Autodesk Inventor part; units mm, degrees
ref_plane "YZ Plane" through (0, 0, 0) normal (1, 0, 0) x (0, 1, 0)
ref_plane "XZ Plane" through (0, 0, 0) normal (0, 1, 0) x (-1, 0, 0)
ref_plane "XY Plane" through (0, 0, 0) normal (0, 0, 1) x (1, 0, 0)
sketch "Sketch1" plane through (0, 0, 0) normal (0, 0, 1) x (1, 0, 0)
  line L0 (-1.27, -1.27) -> (1.27, -1.27)
  line L1 (1.27, -1.27) -> (1.27, 1.27)
  line L2 (1.27, 1.27) -> (-1.27, 1.27)
  line L3 (-1.27, 1.27) -> (-1.27, -1.27)
  line L4 (-1.27, -1.27) -> (1.27, 1.27) construction
  line L5 (1.27, -1.27) -> (-1.27, 1.27) construction
  line L6 (-1.07, 1.07) -> (1.07, 1.07)
  line L7 (1.07, 1.07) -> (1.07, -1.07)
  line L8 (1.07, -1.07) -> (-1.07, -1.07)
  line L9 (-1.07, -1.07) -> (-1.07, 1.07)
  point P0 (0, 0)
  point P1 (0, 1.07)
  dimension "d0" = 2.54
  dimension "d1" = 2.54
  dimension "d2" = 0.2
extrude "Extrusion1" add sketch "Sketch1" along normal blind 8.3 contours L3 L2 L1 L0 | L6 L7 L8 L9
shell "Shell1" thickness 0.4 removed faces 1 at (0.4233, -0.4233, 0)
chamfer "Chamfer1" distance 0.4 angle 45 4 edges at (0, -0.87, 0) (-0.87, 0, 0) (0, 0.87, 0) (0.87, 0, 0)
pattern_linear "Rectangular Pattern1" count 8 spacing 2.54 along (1, 0, 0)
properties part number "CasePinos"
Could you check a few things on this model? Use its own coordinates, in mm. Coordinates: 2 decimals unless noted, no trailing zeros. Answer in a Markdown table with one row per item.
(1) Imagine slicing it at B-B (z = 1.25). Give the number of separate pieces and of enclosed holes in the cut face, plus the area to 3 significant figures.
Results found:
| item | result |
|---|---|
| separate pieces | 1 |
| enclosed holes | 8 |
| area | 27.4 mm^2 |
(2) If I drill on probe 1 along Y at (x, z) = (2.75, 4); probe 2 along Z at (x, y) = (17, -0.3); probe 3 along Z at (x, y) = (5.5, 1.1), over which ranges is the centre line in solid material (lowest first)?
Results found:
| item | result |
|---|---|
| probe 1 | y = -1.27 to -0.87, 0.87 to 1.27 |
| probe 2 | z = 7.9 to 8.3 |
| probe 3 | z = 0.17 to 8.3 |
(3) Thinking about a two-plate mould opening in X: for faces 1 (the face through (9, 1.27, 4)), 2 (the face through (5, 0, 7.9)), 3 (the face through (-1.27, 0, 4)), which applies, released by +X, released by -X, zero draft, split by the parting line, or undercut?
Results found:
| item | result |
|---|---|
| face 1 | zero draft |
| face 2 | undercut |
| face 3 | released by -X |
(4) Will these pins go through, and if not, where does the flat tip stop? pin 1 Ø0.5 at (x, y) = (7.5, 0) entering from -Z; pin 2 Ø1.4 at (x, y) = (13, 0) entering from -Z.
Results found:
| item | result |
|---|---|
| pin 1 | stops at z = 7.9 |
| pin 2 | stops at z = 0.27 |
